Read the model definition and answer for the solid it produces. Units are mm, in the model's axes. Face numbers are marked on the shaded views. A direction names the side the tool comes from. Give positions to 0.01 mm unless a question says otherwise; leave off trailing zeros. Order: outer loops, then holes, each group sorted by start corner. A loop starts at its lowest first (then second) coordinate and runs counter-clockwise, first axis right, second up.
Item 1: A cutting plane is placed at A-A (x = -21). Write down the section's boundary in (y, z), plus the area to 3 significant figures.
Item 2: A cutting plane is placed at B-B (x = 0). Write down the section's boundary in (y, z).
Item 3: The mould has two halves that part along X. Classify the marked faces 3, 4 and 5: +X half, -X half, draft (parallel to the pull), parting line (faces both ways), or undercut.
Item 4: Find the intervals of material crossed by line 1 along Y through (x, z) = (0, -6); line 2 along Z through (x, y) = (25.5, 0); line 3 along Y through (x, z) = (0, 13.5), in increasing order.
Item 5: Which of the six approach directions +Z, -Z, +X, -X, +Y, -Y give full straight-line access (tool end or side, diameter ignored) to the marked faces 1 and 2?
Item 6: A cutting plane is placed at D-D (z = -3.5). Write down the section's boundary in (x, y).
Item 7: A cutting plane is placed at C-C (y = 0). State how many separate pieces and enclosed holes the cut face has, plus the area to 3 significant figures.
Item 8: Given pin 1 Ø0.6 at (x, z) = (-21.5, -8.5) entering from +Y; pin 2 Ø0.9 at (x, z) = (18, 18.5) entering from -Y; pin 3 Ø2 at (x, z) = (18.5, 14.5) entering from +Y, each flat-ended and moving along its own axis, determine where each tip first touches the part or whether it passes through.
from build123d import *

# Parameters (mm, degrees)
SKETCH_1_R          = 19
EXTRUDE_1_DEPTH     = 20
EXTRUDE_2_DEPTH     = 3
SKETCH_6_R          = 17
CUT_EXTRUDE_1_DEPTH = 18
SKETCH_7_R          = 17
SKETCH_7_R_2        = 15
EXTRUDE_3_DEPTH     = 9.5
CUT_EXTRUDE_2_REACH = 44.629
SKETCH_8_R          = 13
EXTRUDE_START       = -2
EXTRUDE_4_DEPTH     = 2
CUT_EXTRUDE_3_REACH = 49.828
SKETCH_14_R         = 1
CUT_EXTRUDE_4_REACH = 48.038
SKETCH_15_R         = 1.5


with BuildPart() as part:
    # 草图1 → 凸台-拉伸1 (new body)
    with BuildSketch(Plane.XY):
        Circle(SKETCH_1_R)
    extrude(amount=EXTRUDE_1_DEPTH)

    # 草图3 → 凸台-拉伸2 (add)
    with BuildSketch(Plane.XY.offset(20)):
        with BuildLine():
            Line((-22.5, 10), (22.5, 10))
            ThreePointArc((22.5, 10), (32.5, 0), (22.5, -10))
            Line((22.5, -10), (-22.5, -10))
            ThreePointArc((-22.5, -10), (-32.5, 0), (-22.5, 10))
        make_face()
    extrude(amount=-EXTRUDE_2_DEPTH)

    # 草图6 → 切除-拉伸1 (cut)
    with BuildSketch(Plane.XY.offset(20)):
        Circle(SKETCH_6_R)
    extrude(amount=-CUT_EXTRUDE_1_DEPTH, mode=Mode.SUBTRACT)

    # 草图7 → 凸台-拉伸3 (add)
    with BuildSketch(Plane(origin=(0, 0, 0), x_dir=(-1, 0, 0), z_dir=(0, 0, -1))):
        with Locations(Location((0, 0, 0), (0, 0, 180))):
            Circle(SKETCH_7_R)
        Circle(SKETCH_7_R_2, mode=Mode.SUBTRACT)
    extrude(amount=EXTRUDE_3_DEPTH)

    # 草图8 → 切除-拉伸2 (cut, up to next)
    with BuildSketch(Plane(origin=(0, 0, 0), x_dir=(-1, 0, 0), z_dir=(0, 0, -1)), mode=Mode.PRIVATE) as cut_extrude_2_sk1:
        Circle(SKETCH_8_R)
    cut_extrude_2_tool1 = extrude(cut_extrude_2_sk1.sketch, amount=-CUT_EXTRUDE_2_REACH, mode=Mode.PRIVATE) & part.part
    add(cut_extrude_2_tool1.solids().sort_by_distance((0, 0, 0))[0], mode=Mode.SUBTRACT)

    # 草图10 → 凸台-拉伸4 (add)
    with BuildSketch(Plane(origin=(0, 0, -9.5), x_dir=(-1, 0, 0), z_dir=(0, 0, -1)).offset(EXTRUDE_START)):
        with BuildLine():
            Line((-16.815171721, 2.5), (-23.815171721, 2.5))
            ThreePointArc((-23.815171721, 2.5), (-26.315171721, 0), (-23.815171721, -2.5))
            Line((-23.815171721, -2.5), (-16.815171721, -2.5))
            ThreePointArc((-16.815171721, -2.5), (-17, 0), (-16.815171721, 2.5))
        make_face()
        with BuildLine():
            Line((16.815171721, 2.5), (23.815171721, 2.5))
            ThreePointArc((23.815171721, 2.5), (26.315171721, 0), (23.815171721, -2.5))
            Line((23.815171721, -2.5), (16.815171721, -2.5))
            ThreePointArc((16.815171721, -2.5), (17, 0), (16.815171721, 2.5))
        make_face()
    extrude(amount=EXTRUDE_4_DEPTH)

    # 草图14 → 切除-拉伸3 (cut, up to next)
    with BuildSketch(Plane(origin=(0, 0, -9.5), x_dir=(-1, 0, 0), z_dir=(0, 0, -1)), mode=Mode.PRIVATE) as cut_extrude_3_sk1:
        with Locations((-23.815171721, 0)):
            Circle(SKETCH_14_R)
    cut_extrude_3_tool1 = extrude(cut_extrude_3_sk1.sketch, amount=-CUT_EXTRUDE_3_REACH, mode=Mode.PRIVATE) & part.part
    cut_extrude_3 = cut_extrude_3_tool1.solids().sort_by_distance((23.815172, 0, -9.5))[0]
    add(cut_extrude_3, mode=Mode.SUBTRACT)

    # 草图15 → 切除-拉伸4 (cut, up to next)
    with BuildSketch(Plane(origin=(0, 0, 17), x_dir=(-1, 0, 0), z_dir=(0, 0, -1)), mode=Mode.PRIVATE) as cut_extrude_4_sk1:
        with Locations((-23.815171721, 0)):
            Circle(SKETCH_15_R)
    cut_extrude_4_tool1 = extrude(cut_extrude_4_sk1.sketch, amount=-CUT_EXTRUDE_4_REACH, mode=Mode.PRIVATE) & part.part
    cut_extrude_4 = cut_extrude_4_tool1.solids().sort_by_distance((23.815172, 0, 17))[0]
    add(cut_extrude_4, mode=Mode.SUBTRACT)

    # 镜向1: 切除-拉伸3, 切除-拉伸4 across plane
    add(cut_extrude_3.mirror(Plane(origin=(0, 0, 0), x_dir=(0, 0, 1), z_dir=(1, 0, 0))), mode=Mode.SUBTRACT)
    add(cut_extrude_4.mirror(Plane(origin=(0, 0, 0), x_dir=(0, 0, 1), z_dir=(1, 0, 0))), mode=Mode.SUBTRACT)


solid = part.part
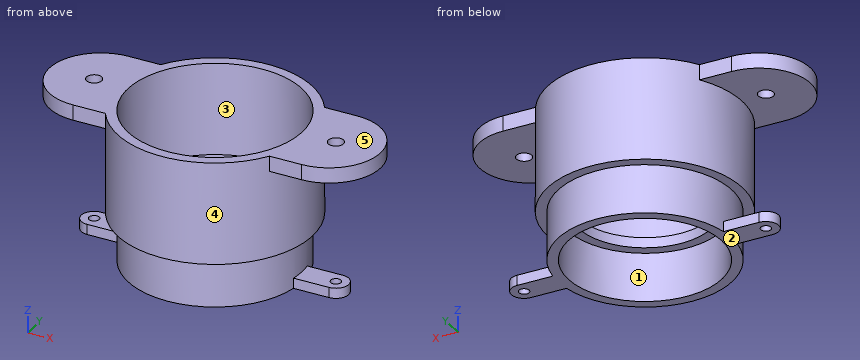
Response values:
1. outline: (-10, 17) - (10, 17) - (10, 20) - (-10, 20) - close; (-2.5, -9.5) - (2.5, -9.5) - (2.5, -7.5) - (-2.5, -7.5) - close
1. area: 70.0 mm2
2. outline: (-19, 0) - (-17, 0) - (-17, -9.5) - (-15, -9.5) - (-15, 0) - (-13, 0) - (-13, 2) - (-17, 2) - (-17, 20) - (-19, 20) - close; (13, 0) - (15, 0) - (15, -9.5) - (17, -9.5) - (17, 0) - (19, 0) - (19, 20) - (17, 20) - (17, 2) - (13, 2) - close
3. face 3: undercut
3. face 4: parting line
3. face 5: draft
4. line 1: y = -17 to -15, 15 to 17
4. line 2: z = -9.5 to -7.5, 17 to 20
4. line 3: y = -19 to -17, 17 to 19
5. face 1: -Z
5. face 2: -Z, +X, -X, +Y, -Y
6. outline: circle Ø34 at (0, 0); hole circle Ø30 at (0, 0)
7. separate pieces: 6
7. enclosed holes: 0
7. area: 226 mm2
8. pin 1: stops at y = 2.5
8. pin 2: stops at y = -10
8. pin 3: stops at y = 7.4
